```python
from build123d import *

# Parameters (mm, degrees)
F0_W     = 3
F0_H     = 12.5
F1_DEPTH = 80
F3_D     = 5
F4_R     = 5


with BuildPart() as f1:
    # F0 (on Top) → F1 (new body)
    with BuildSketch(Plane.XY):
        Rectangle(F0_W, F0_H)
    extrude(amount=F1_DEPTH)

    # F3 (through all)
    with Locations(Plane(origin=(-1.5, 0, 0), x_dir=(0, -1, 0), z_dir=(-1, 0, 0))):
        with Locations((0, 75), (0, 5)):
            Hole(F3_D / 2)

    # F4
    f4_edges = [f1.edges().sort_by_distance(p)[0] for p in [
        (0, -6.25, 80),
        (0, 6.25, 80),
        (0, 6.25, 0),
        (0, -6.25, 0),
    ]]
    fillet(f4_edges, radius=F4_R)


solid = f1.part
```
Verification items for the finished model (mm, model axes). Coordinates: 2 decimals unless noted, no trailing zeros. Loops run counter-clockwise (first coordinate to the right, second up) from the corner with the lowest first, then second, coordinate; pieces in that order, holes last. Notation, with made-up numbers: (24.25, 79) -> (34.25, 79) arc R26 ccw to (34.25, 109) -> close; hole circle Ø5 at (84, -20.75). An arc over 180 degrees is marked (long way). Answer in a Markdown table with one row per item. Add a question column.
1. Section check A-A, the plane x = -0.2. Enter the section's corners in (y, z), then the cut area to 3 significant figures.
2. Material ranges on probe 1 along Z at (x, y) = (-0.4, 0); probe 2 along Z at (x, y) = (0.8, -1.25); probe 3 along Y at (x, z) = (-0.9, 73.5), recorded low to high. Write a range as [from, to].
3. Draft check along Z on faces 1 (the face through (1.5, 0, 39)), 2 (the face through (0.02, -0.54, 72.56)), 3 (the face through (0.02, -4.82, 78.5)). Enter one of: +Z half, -Z half, draft (parallel to the pull), parting line (faces both ways), or undercut.
4. Section check B-B, the plane y = 4.25. Enter the section's corners in (x, z), then the cut area to 3 significant figures.
5. Depth check by flat-ended pin: P1, Ø3, axis at y = 0, z = 5, coming from the -X side. Enter the tip coordinate at first touch or a pass-through.
Derived:
| question | item | result |
|---|---|---|
| 1 | outline | (-6.25, 5) arc R5 ccw to (-1.25, 0) -> (1.25, 0) arc R5 ccw to (6.25, 5) -> (6.25, 75) arc R5 ccw to (1.25, 80) -> (-1.25, 80) arc R5 ccw to (-6.25, 75) -> close; hole circle Ø5 at (0, 5); hole circle Ø5 at (0, 75) |
| 1 | area | 939 mm² |
| 2 | probe 1 | z = [0, 2.5], [7.5, 72.5], [77.5, 80] |
| 2 | probe 2 | z = [0, 2.83], [7.17, 72.83], [77.17, 80] |
| 2 | probe 3 | y = [-6.25, -2], [2, 6.25] |
| 3 | face 1 | draft |
| 3 | face 2 | undercut |
| 3 | face 3 | +Z half |
| 4 | outline | (-1.5, 1) -> (1.5, 1) -> (1.5, 79) -> (-1.5, 79) -> close |
| 4 | area | 234 mm² |
| 5 | P1 | passes through |
